The listing builds one solid part. Answer for the finished solid, in the listing's coordinates (mm). Give positions to 0.01 mm unless a question says otherwise; leave off trailing zeros. Order: outer loops, then holes, each group sorted by start corner. A loop starts at its lowest first (then second) coordinate and runs counter-clockwise, first axis right, second up. Notation, with made-up numbers: (67, -9.5) -> (102, -9.5) arc R30 ccw to (102, 24.5) -> close; hole circle Ø8 at (-21.5, 81). An arc over 180 degrees is marked (long way). Write item = value, one per line. Start each with the question number.
```python
from build123d import *

# Parameters (mm, degrees)
SKETCH1_W           = 500
SKETCH1_H           = 200
BOSS_EXTRUDE1_DEPTH = 3.175
SKETCH2_W           = 50.5
SKETCH2_H           = 6.6
CUT_EXTRUDE1_DEPTH  = 270.333106951
LPATTERN1_COUNT     = 5
LPATTERN1_PITCH     = 100
SKETCH3_W           = 6.6
SKETCH3_H           = 56.15
SKETCH3_H_2         = 62.75
SKETCH3_H_3         = 75
CUT_EXTRUDE2_DEPTH  = 270.333106951
SKETCH4_R           = 4
AXLE_HOLES_DEPTH    = 270.333106951


with BuildPart() as part:
    # Sketch1 → Boss-Extrude1 (new, symmetric)
    with BuildSketch(Plane(origin=(0, 0, 0), x_dir=(1, 0, 0), z_dir=(0, 1, 0))):
        Rectangle(SKETCH1_W, SKETCH1_H)
    extrude(amount=BOSS_EXTRUDE1_DEPTH, both=True)

    # Sketch2 → Cut-Extrude1 (cut, through all)
    with BuildSketch(Plane(origin=(0, 3.175, 0), x_dir=(1, 0, 0), z_dir=(0, 1, 0))):
        with Locations((-175, -96.7)):
            Rectangle(SKETCH2_W, SKETCH2_H)
    cut_extrude1 = extrude(amount=-CUT_EXTRUDE1_DEPTH, mode=Mode.SUBTRACT)

    # LPattern1: Cut-Extrude1 ×5
    with Locations(*[(i * LPATTERN1_PITCH, 0, 0) for i in range(1, LPATTERN1_COUNT)]):
        add(cut_extrude1, mode=Mode.SUBTRACT)

    # Sketch3 → Cut-Extrude2 (cut, through all)
    with BuildSketch(Plane(origin=(0, 3.175, 0), x_dir=(1, 0, 0), z_dir=(0, 1, 0))):
        with Locations((246.7, -65.325)):
            Rectangle(SKETCH3_W, SKETCH3_H)
        with Locations((246.7, 68.625)):
            Rectangle(SKETCH3_W, SKETCH3_H_2)
        with Locations((-246.7, 0)):
            Rectangle(SKETCH3_W, SKETCH3_H_3)
    extrude(amount=-CUT_EXTRUDE2_DEPTH, mode=Mode.SUBTRACT)

    # Sketch4 → Axle Holes (cut, through all)
    with BuildSketch(Plane(origin=(0, 3.175, 0), x_dir=(1, 0, 0), z_dir=(0, 1, 0))):
        with Locations(Location((-200, -20, 0), (0, 0, 270))):
            Circle(SKETCH4_R)
        with Locations(Location((200, -20, 0), (0, 0, 270))):
            Circle(SKETCH4_R)
    extrude(amount=-AXLE_HOLES_DEPTH, mode=Mode.SUBTRACT)


solid = part.part
```
Item 1: A cutting plane is placed at A-A, the plane y = 0.5. Count the separate pieces of the cut face and the enclosed holes in it, plus the area to 3 significant figures.
Item 2: A cutting plane is placed at B-B, the plane x = -68. Write down the section's boundary in (y, z) (3 decimals).
Item 3: Consider L1, parallel to X at y = -1.5, z = 20; L2, parallel to X at y = 0.25, z = 90; L3, parallel to X at y = 2.5, z = 14. Determine where each line is inside the solid, lowest interval first. Write a range as from..to.
Item 4: Flat-ended cylindrical pins translate along their axes: pin 1 (3 mm diameter, centred on y = -1.5, z = 95, fed in from +X); pin 2 (3 mm diameter, centred on y = 0.5, z = 16, fed in from -X); pin 3 (3 mm diameter, centred on y = 1, z = -83, fed in from +X). Find the tip coordinate at first contact, or state that the pin passes through.
Check values:
q1.separate_pieces = 1
q1.enclosed_holes = 2
q1.area = 97,000 mm^2
q2.outline = (-3.175, -100) -> (3.175, -100) -> (3.175, 93.4) -> (-3.175, 93.4) -> close
q3.L1 = -243.4..-204, -196..196, 204..250
q3.L2 = -250..243.4
q3.L3 = -243.4..250
q4.pin_1 = 199.75
q4.pin_2 = -243.4
q4.pin_3 = 243.4
